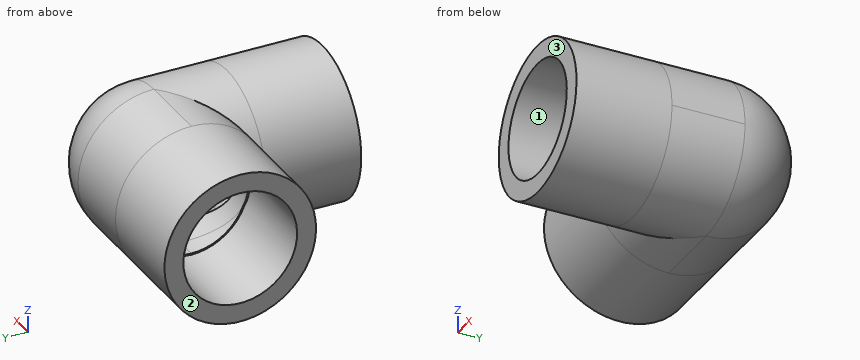
```python
from build123d import *
from build123d.topology import SkipClean

# Parameters (mm, degrees)
SKETCH1_W    = 13.493749999999999
SKETCH1_H    = 2.676524999999998
SWEEP2_ANGLE = 180
SKETCH12_R   = 7.861299999999998
SKETCH12_2_R = 7.861299999999998
SKETCH16_R   = 7.861299999999998
SKETCH16_2_R = 7.861299999999998


# Read off the part's stored shape, not the designer's step: Sweep2
with BuildPart() as part:
    # Sketch1 → Revolve1 (revolve)
    with BuildSketch(Plane.XY, mode=Mode.PRIVATE) as revolve1_sk:
        with Locations((-17.065625, 9.3773625)):
            Rectangle(SKETCH1_W, SKETCH1_H)
    revolve(revolve1_sk.sketch.rotate(Axis((-34.18819835941514, 0, 0), (1, 0, 0)), 90), axis=Axis((-34.18819835941514, 0, 0), (1, 0, 0)))

    # Sketch2 → Revolve2 (revolve)
    with BuildSketch(Plane.XY, mode=Mode.PRIVATE) as revolve2_sk:
        Polygon((8.039100000000003, -10.31875), (10.715625000000001, -10.31875), (10.715625000000003, -23.8125), (8.039100000000003, -23.8125), align=None)
    revolve(revolve2_sk.sketch.rotate(Axis((0, 0, 0), (0, -1, 0)), 90), axis=Axis((0, 0, 0), (0, -1, 0)))

    # Sweep2 outline → Sweep2 (revolve)
    with SkipClean():  # the faces are left unmerged after this step: merging them gives an invalid solid
        with BuildSketch(Plane(origin=(0, 0, 0), x_dir=(0, 6e-17, -1), z_dir=(0, -1, -6e-17))):
            with BuildLine():
                Line((10.715625, -10.31875), (10.715625, 0))
                ThreePointArc((10.715625, 0), (7.577091102, 7.577091102), (0, 10.715625))
                Line((0, 10.715625), (0, 7.8613))
                ThreePointArc((0, 7.8613), (5.558778539, 5.558778539), (7.8613, 0))
                Line((7.8613, 0), (7.8613, -10.31875))
                Line((7.8613, -10.31875), (10.715625, -10.31875))
            make_face()
        revolve(axis=Axis((0, 0, 0), (1, 0, 0)), revolution_arc=SWEEP2_ANGLE)

    # Sweep3: sweep along a path in Sketch9
    with SkipClean():  # the faces are left unmerged after this step: merging them gives an invalid solid
        with BuildLine(Plane.XZ) as sweep3_path:
            CenterArc((0, 0), 10.715625, 0, 360)
        # Sketch8 → Sweep3 (sweep)
        with BuildSketch(Plane(origin=(0, 0, 0), x_dir=(0, 0, -1), z_dir=(1, 0, 0))):
            Polygon((-10.715625000000003, 7e-17), (-7.861299999999998, 0), (-7.861299999999998, -10.318750000000001), (-10.715625000000003, -10.318750000000001), align=None)
        sweep(path=sweep3_path.line)

    # Sweep4: sweep along a path in Sketch10
    with BuildLine(Plane(origin=(-10.318750000000001, 0, 0), x_dir=(0, 0, -1), z_dir=(1, 0, 0))) as sweep4_path:
        ThreePointArc((-10.715625, -3.87e-15), (6.6e-16, -10.715625), (10.715625, -3.87e-15))
    # Sketch11 → Sweep4 (sweep)
    with BuildSketch(Plane.XZ):
        Polygon((-10.318750000000001, 10.715625), (1.19e-15, 10.715625), (1.54e-15, 7.861299999999998), (-10.318750000000001, 7.861299999999998), align=None)
    sweep(path=sweep4_path.line)

    # Cut-Sweep3: sweep along a path in Sketch14
    with BuildLine(Plane.XY) as cut_sweep3_path:
        Line((1.73e-15, 8.039100000000001), (-10.318750000000001, 8.0391))
    # Sketch12 → Cut-Sweep3 (sweep, cut)
    with BuildSketch(Plane.ZY.offset(10.318750000000001)):
        Circle(SKETCH12_R)
    sweep(path=cut_sweep3_path.line, mode=Mode.SUBTRACT)

    # Cut-Sweep4: sweep along a path in Sketch15
    with BuildLine(Plane.XY) as cut_sweep4_path:
        Line((-10.318750000000001, 5.616092889966187), (-23.8125, 5.616092889966185))
    # Sketch12<2> → Cut-Sweep4 (sweep, cut)
    with BuildSketch(Plane.ZY.offset(10.318750000000001)):
        Circle(SKETCH12_2_R)
    sweep(path=cut_sweep4_path.line, mode=Mode.SUBTRACT)

    # Cut-Sweep6: sweep along a path in Sketch17
    with BuildLine(Plane.XY) as cut_sweep6_path:
        Line((7.861299999999998, 0), (7.861299999999998, -10.318750000000001))
    # Sketch16 → Cut-Sweep6 (sweep, cut)
    with BuildSketch(Plane.XZ.offset(10.318750000000001)):
        Circle(SKETCH16_R)
    sweep(path=cut_sweep6_path.line, mode=Mode.SUBTRACT)

    # Cut-Sweep7: sweep along a path in Sketch18
    with BuildLine(Plane.XY) as cut_sweep7_path:
        Line((-7.861299999999989, -10.318750000000001), (-7.8612999999999875, -23.8125))
    # Sketch16<2> → Cut-Sweep7 (sweep, cut)
    with BuildSketch(Plane.XZ.offset(10.318750000000001)):
        Circle(SKETCH16_2_R)
    sweep(path=cut_sweep7_path.line, mode=Mode.SUBTRACT)


solid = part.part
```
Build history of the part. All positions in model axes, mm. Face numbers are marked on the shaded views. Coordinates: 2 decimals unless noted, no trailing zeros. Order: outer loops, then holes, each group sorted by start corner. A loop starts at its lowest first (then second) coordinate and runs counter-clockwise, first axis right, second up. Notation, with made-up numbers: M 6,-25.5 L 59,-25.5 A20 ccw 59,10.5 Z; hole C 89.5,64.5 d9. An arc over 180 degrees is marked long. One line per question, with ' | ' between items. Start each with the question number.
1. Cut at D-D (x = -9). Write the cut outline in (y, z), plus the area to 3 significant figures.
2. Flat gauge pins, fed straight in: P1, Ø3, axis at x = 2, y = -7, coming from the -Z side; P2, Ø12, axis at x = -14.5, y = -12.5, coming from the +Z side; P3, Ø4, axis at y = -16, z = 4.5, coming from the -X side. Where does each tip first touch, or does it go through?
3. Mould opens along X. For the marked faces 1, 2 and 3 say: +X half, -X half, draft (parallel to the pull), parting line (faces both ways), or undercut.
4. Wall check: line 1 along X through (y, z) = (-14.75, 0); line 2 along X through (y, z) = (-5, 7.25); line 3 along Y through (x, z) = (-17, -5.75). Give the ranges that are in metal, low to high. Write a range as [from, to].
5. Cut at C-C (y = 3.5). Write the cut outline in (x, z), plus the area to 3 significant figures.
6. Cut at A-A (x = -19). Write the cut outline in (y, z), plus the area to 3 significant figures.
The answers:
1) outline: M -23.81,-5.82 L -9,-5.82 A10.72 ccw long -9,5.82 L -23.81,5.82 Z; hole C 0,0 d15.72 | area: 325 mm2
2) P1: stops at z = -10.7 | P2: stops at z = 8.52 | P3: stops at x = -10.42
3) face 1: undercut | face 2: -X half | face 3: draft
4) line 1: x = [-10.72, -8.04], [8.04, 10.72] | line 2: x = [-23.81, -3.04], [3.04, 7.89] | line 3: y = [-9.04, -5.62], [5.62, 9.04]
5) outline: M -23.81,-10.13 L 0,-10.13 A10.13 ccw 0,10.13 L -23.81,10.13 L -23.81,7.24 L -10.32,7.24 L -10.32,7.04 L 0,7.04 A7.04 cw 0,-7.04 L -10.32,-7.04 L -10.32,-7.24 L -23.81,-7.24 Z | area: 225 mm2
6) outline: C 0,0 d21.43; hole C 0,0 d16.08 | area: 158 mm2
